```python
from build123d import *

# Parameters (mm, degrees)
SKETCH_1_W             = 150
SKETCH_1_H             = 205
SM_BASE_FLANGE_1_DEPTH = 20
CHAMFER_1_SIZE         = 16
CHAMFER_1_SIZE2        = 11.203320611
CHAMFER_2_SIZE         = 16
CHAMFER_2_SIZE2        = 11.203320611


# Sheet-metal steps are written as plain solids
with BuildPart() as part:
    # Sketch 1 → 基体-法兰1 (new body)
    with BuildSketch(Plane.XY):
        Rectangle(SKETCH_1_W, SKETCH_1_H)
    extrude(amount=-SM_BASE_FLANGE_1_DEPTH)

    # 倒角1
    chamfer_1_edges = [part.edges().sort_by_distance(p)[0] for p in [
        (0, 102.5, -20),
    ]]
    chamfer_1_side = [part.faces().sort_by_distance(p)[0] for p in [
        (0, 102.5, -10),
    ]]
    chamfer(chamfer_1_edges, length=CHAMFER_1_SIZE, length2=CHAMFER_1_SIZE2, reference=chamfer_1_side[0])

    # 倒角2
    chamfer_2_edges = [part.edges().sort_by_distance(p)[0] for p in [
        (0, -102.5, -20),
    ]]
    chamfer_2_side = [part.faces().sort_by_distance(p)[0] for p in [
        (0, -102.5, -10),
    ]]
    chamfer(chamfer_2_edges, length=CHAMFER_2_SIZE, length2=CHAMFER_2_SIZE2, reference=chamfer_2_side[0])


solid = part.part
```
Work out the finished part from the listing and answer in its coordinate system (mm). Round coordinates to 2 decimals unless told otherwise and drop trailing zeros. Write each loop counter-clockwise with the first axis right and the second up, starting at its lowest first coordinate (ties: lowest second). Pieces come first, ordered by that corner, then holes.
1) Consider probe 1 along Y at (x, z) = (-31, -14); probe 2 along Y at (x, z) = (57, -10). Determine where each line is inside the solid, lowest interval first.
2) A cutting plane is placed at B-B on z = -10.25. Determine the outline of the cut face in (x, y).
3) Flat-ended cylindrical pins translate along their axes: P1, Ø10, axis at x = -37.5, z = -10, coming from the -Y side; P2, Ø5, axis at x = 27.5, z = -9.5, coming from the +Y side. Find the tip coordinate at first contact, or state that the pin passes through.
4) A cutting plane is placed at A-A on x = 33. Determine the outline of the cut face in (y, z), and give its area (3 significant figures).
Entries:
1. probe 1: y = -95.5 to 95.5
1. probe 2: y = -98.3 to 98.3
2. outline: (-75, -98.12) - (75, -98.12) - (75, 98.12) - (-75, 98.12) - close
3. P1: stops at y = -101.8
3. P2: stops at y = 100.4
4. outline: (-102.5, -4) - (-91.3, -20) - (91.3, -20) - (102.5, -4) - (102.5, 0) - (-102.5, 0) - close
4. area: 3,920 mm2
